```python
from build123d import *

# Parameters (mm, degrees)
F0_W     = 21.43125
F0_H     = 21.43125
F0_R     = 2.38125
F1_DEPTH = 3.175
F3_DEPTH = 18.25625


# Not quite as in the source:
# - a length typed as a fraction of an inch, garbled in the dataset ("3 / 203.2 mm" for 3/8 in), is restored


with BuildPart() as f1:
    # F0 (on Top) → F1 (new body)
    with BuildSketch(Plane.XY):
        Rectangle(F0_W, F0_H)
        Circle(F0_R, mode=Mode.SUBTRACT)
        Polygon((32.146875, -10.715625), (10.715625, 10.715625), (10.715625, -10.715625), align=None)
    extrude(amount=F1_DEPTH)

    # F2 (on face) → F3 (join)
    with BuildSketch(Plane.XY.offset(3.175)):
        Polygon((32.146875, -10.715625), (10.715625, 10.715625), (8.4705609697, 8.4705609697), (27.6567469395, -10.715625), align=None)
        Polygon((8.4705609697, 8.4705609697), (10.715625, 10.715625), (6.2254969395, 10.715625), align=None)
    extrude(amount=F3_DEPTH)


solid = f1.part
```
Source: CAD feature listing. Evaluate the final solid. Frame: model axes, mm. A direction names the side the tool comes from. Give positions to 0.01 mm unless a question says otherwise; leave off trailing zeros. Loops run counter-clockwise (first coordinate to the right, second up) from the corner with the lowest first, then second, coordinate; pieces in that order, holes last. Notation, with made-up numbers: (82, -12) -> (126, -12) arc R11 cw to (126, 9) -> close; hole circle Ø3 at (-36.75, 36.5). An arc over 180 degrees is marked (long way). Put each result on its own line as item: value. Start each with the question number.
1) Cut plane D-D (x = -7). Return loops of the section in (y, z) (3 decimals).
2) Cut plane C-C (z = 15.75). Return loops of the section in (x, y), then the cut area to 3 significant figures.
3) Cut plane A-A (x = 0). Return loops of the section in (y, z) (3 decimals), then the cut area to 3 significant figures.
4) Contact query for flat-ended pins moving along their axis: P1, Ø7.5, axis at x = 0, y = 0, coming from the +Z side (3 decimals); P2, Ø3, axis at x = 26, z = 16.5, coming from the +Y side; P3, Ø1.5, axis at x = 12, z = 15.5, coming from the -Y side. Output: stop coordinate, or through.
5) Material intervals for probe 1 along Y at (x, z) = (0, 1.25); probe 2 along Z at (x, y) = (6, -5.5) (3 decimals); probe 3 along X at (y, z) = (1.75, 8), sorted ascending.
6) Draft query along Y for faces 3 (the face through (19, -10.716, 2)), 4 (the face through (6, -2, 0)), 5 (the face through (-1.89, -1.45, 1.57)), 6 (the face through (21.58, -0.15, 10.57)). Return one class per face: released by +Y, released by -Y, zero draft, split by the parting line, or undercut.
7) Reachability of faces 1 (the face through (4, -2, 3.175)), 2 (the face through (7, 10.716, 7)) from +Z, -Z, +X, -X, +Y, -Y: full face, straight path, thin tool, end or side. Return the list, or none.
8) Cut plane B-B (y = 0). Return loops of the section in (x, z) (3 decimals), then the cut area to 3 significant figures.
Results are:
1. outline: (-10.716, 0) -> (10.716, 0) -> (10.716, 3.175) -> (-10.716, 3.175) -> close
2. outline: (6.23, 10.72) -> (27.66, -10.72) -> (32.15, -10.72) -> (10.72, 10.72) -> close
2. area: 96.2 mm2
3. outline: (-10.716, 0) -> (-2.381, 0) -> (-2.381, 3.175) -> (-10.716, 3.175) -> close; (2.381, 0) -> (10.716, 0) -> (10.716, 3.175) -> (2.381, 3.175) -> close
3. area: 52.9 mm2
4. P1: stops at z = 3.175
4. P2: stops at y = -3.07
4. P3: stops at y = 4.19
5. probe 1: y = -10.72 to -2.38, 2.38 to 10.72
5. probe 2: z = 0 to 3.175
5. probe 3: x = 15.19 to 19.68
6. face 3: released by -Y
6. face 4: zero draft
6. face 5: undercut
6. face 6: released by +Y
7. face 1: +Z, -X, -Y
7. face 2: +Z, -Z, +X, -X, +Y
8. outline: (-10.716, 0) -> (-2.381, 0) -> (-2.381, 3.175) -> (-10.716, 3.175) -> close; (2.381, 0) -> (21.431, 0) -> (21.431, 21.431) -> (16.941, 21.431) -> (16.941, 3.175) -> (2.381, 3.175) -> close
8. area: 169 mm2
